Geometry: see drawing. Coordinates: mm, zero at the bounding-box minimum. A direction names the side the tool comes from. Give positions to 0.01 mm unless a question says otherwise; leave off trailing zeros. Write each loop counter-clockwise with the first axis right and the second up, starting at its lowest first coordinate (ties: lowest second). Pieces come first, ordered by that corner, then holes. Notation, with made-up numbers: M 48.5,-36 L 99.5,-36 A18 cw 99.5,-20 Z; hole C 66.25,-19 d8. An arc over 180 degrees is marked long. Use CSV: the item, a comma, the result in double quotes. Start each with the question number.
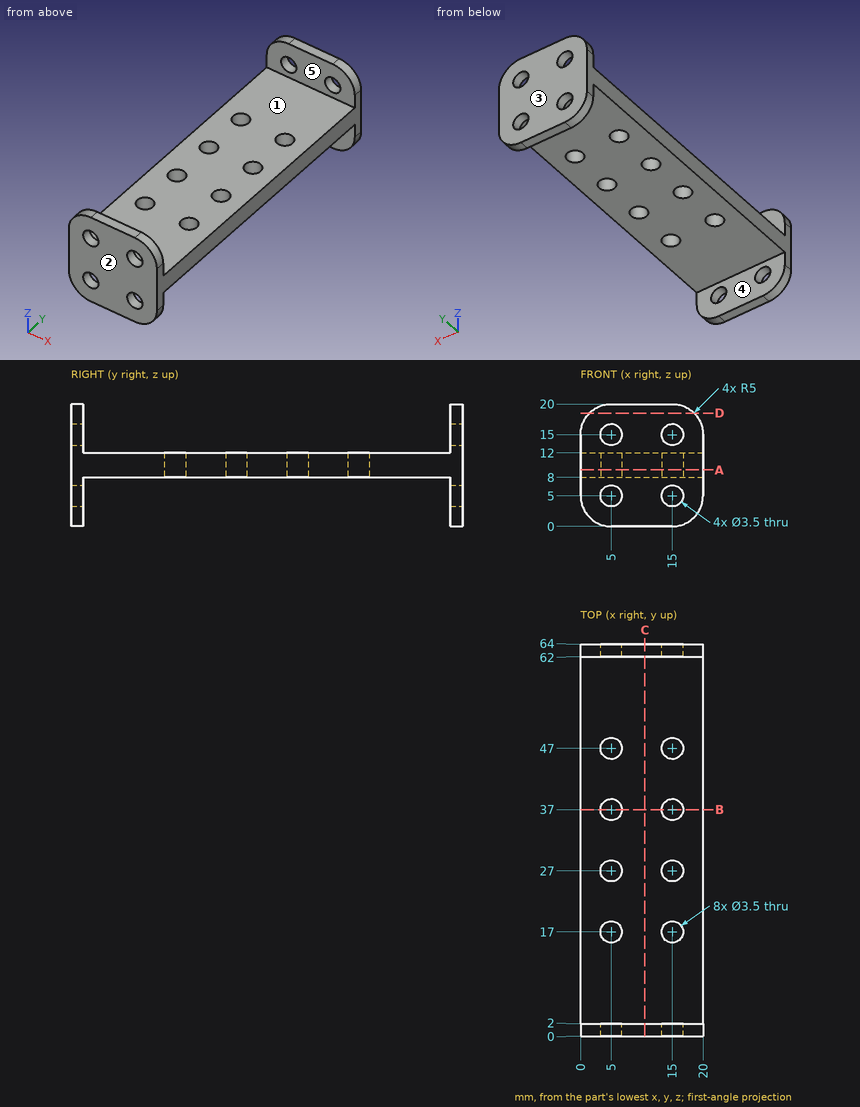
1. First-contact query: pin 1 (6 mm diameter, centred on x = 6, y = 38, fed in from -Z); pin 2 (5.5 mm diameter, centred on x = 5, y = 47, fed in from +Z). Flat tips, straight axial feed; report the tip coordinate or a pass-through.
2. Section A-A on z = 9.25. Give the number of separate pieces and of enclosed holes in the cut face, then the cut area to 3 significant figures.
3. Line query: probe 1 along Z at (x, y) = (5, 63.45); probe 2 along Y at (x, z) = (17.5, 14.5); probe 3 along X at (y, z) = (36, 9). Output: solid intervals per line, ascending.
4. Pull-direction query (Y, two-part tool) for the marked faces 1, 2 and 3; classes: released by +Y, released by -Y, zero draft, split by the parting line, or undercut.
5. Section D-D on z = 18.5. Return loops of the section in (x, y).
6. Section B-B on y = 37. Return loops of the section in (x, z), then the cut area to 3 significant figures.
7. Section C-C on x = 10.5. Return loops of the section in (y, z), then the cut area to 3 significant figures.
8. Access query for the marked faces 4 and 5. Directions: +Z, -Z, +X, -X, +Y, -Y. A direction counts if a zero-diameter tool reaches every point of the face in a straight line with its end or side. Return the directions, or none.
Resolved:
1,pin 1,"stops at z = 8"
1,pin 2,"stops at z = 12"
2,separate pieces,"1"
2,enclosed holes,"8"
2,area,"1,200 mm2"
3,probe 1,"z = 0 to 3.25, 6.75 to 13.25, 16.75 to 20"
3,probe 2,"y = 0 to 2, 62 to 64"
3,probe 3,"x = 0 to 3.56, 6.44 to 13.56, 16.44 to 20"
4,face 1,"undercut"
4,face 2,"released by -Y"
4,face 3,"released by +Y"
5,outline,"M 1.43,0 L 18.57,0 L 18.57,2 L 1.43,2 Z; M 1.43,62 L 18.57,62 L 18.57,64 L 1.43,64 Z"
6,outline,"M 0,8 L 3.25,8 L 3.25,12 L 0,12 Z; M 6.75,8 L 13.25,8 L 13.25,12 L 6.75,12 Z; M 16.75,8 L 20,8 L 20,12 L 16.75,12 Z"
6,area,"52.0 mm2"
7,outline,"M 0,0 L 2,0 L 2,8 L 62,8 L 62,0 L 64,0 L 64,20 L 62,20 L 62,12 L 2,12 L 2,20 L 0,20 Z"
7,area,"320 mm2"
8,face 4,"-Z, +X, -X"
8,face 5,"+Z, +X, -X"
